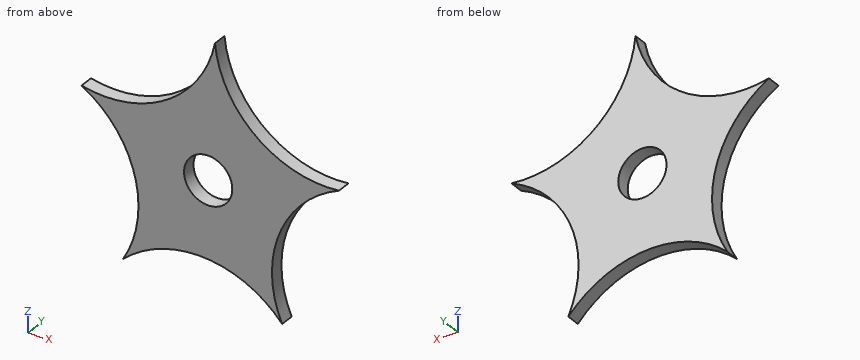
from build123d import *

# Parameters (mm, degrees)
F0_R     = 10.9982
F1_DEPTH = 6.35


with BuildPart() as f1:
    # F0 (on Front) → F1 (new body)
    with BuildSketch(Plane.XZ):
        with BuildLine():
            ThreePointArc((3.120614, 61.683006), (-18.952567, 29.068953), (-57.699702, 22.028977))
            ThreePointArc((-57.699702, 22.028977), (-33.502883, -9.042162), (-38.780991, -48.06835))
            ThreePointArc((-38.780991, -48.06835), (-1.753353, -34.657317), (33.731732, -51.736851))
            ThreePointArc((33.731732, -51.736851), (32.419251, -12.377238), (59.628348, 16.093217))
            ThreePointArc((59.628348, 16.093217), (21.789552, 27.007763), (3.120614, 61.683006))
        make_face()
        Circle(F0_R, mode=Mode.SUBTRACT)
    extrude(amount=F1_DEPTH)


solid = f1.part
Input: part model. Units: mm. Frame: model coordinates. Coordinates: 2 decimals unless noted, no trailing zeros. Loops run counter-clockwise (first coordinate to the right, second up) from the corner with the lowest first, then second, coordinate; pieces in that order, holes last.
(1) Section C-C on z = 29. Return the cut outline in (x, y).
(2) First-contact query: pin 1 Ø2 at (y, z) = (-4, 49.5) entering from +X; pin 2 Ø2 at (y, z) = (-4, 8) entering from -X. Flat tips, straight axial feed; report the tip coordinate or a pass-through.
(3) Section D-D on z = -21.5. Return the cut outline in (x, y), then the cut area to 3 significant figures.
(4) Section B-B on x = 32. Return the cut outline in (y, z), then the cut area to 3 significant figures.
(5) Section A-A on z = 4.5. Return the cut outline in (x, y), then the cut area to 3 significant figures.
(6) Material intervals for probe 1 along Z at (x, y) = (0, -2); probe 2 along X at (y, z) = (-3.5, -3); probe 3 along Z at (x, y) = (7.5, -0.75), sorted ascending.
Data:
1. outline: (-19.06, -6.35) - (19.47, -6.35) - (19.47, 0) - (-19.06, 0) - close
2. pin 1: stops at x = 6.2
2. pin 2: stops at x = -42.52
3. outline: (-31.75, -6.35) - (29.88, -6.35) - (29.88, 0) - (-31.75, 0) - close
3. area: 391 mm2
4. outline: (-6.35, -49.87) - (0, -49.87) - (0, -47.48) - (-6.35, -47.48) - close; (-6.35, -13.52) - (0, -13.52) - (0, 20.61) - (-6.35, 20.61) - close
4. area: 232 mm2
5. outline: (-39.38, -6.35) - (-10.04, -6.35) - (-10.04, 0) - (-39.38, 0) - close; (10.04, -6.35) - (43.06, -6.35) - (43.06, 0) - (10.04, 0) - close
5. area: 396 mm2
6. probe 1: z = -34.78 to -11, 11 to 51.62
6. probe 2: x = -35.55 to -10.58, 10.58 to 37.16
6. probe 3: z = -35.99 to -8.04, 8.04 to 45.39
